```python
from build123d import *

# Parameters (mm, degrees)
SHELL1_T = -0.75


with BuildPart() as part:
    # Sketch1 → Revolve1 (revolve)
    with BuildSketch(Plane(origin=(0, 0, 0), x_dir=(1, 0, 0), z_dir=(0, 1, 0)), mode=Mode.PRIVATE) as revolve1_sk:
        Polygon((3.5, 16.5), (3.5, -16.5), (2.5, -16.5), (2.5, -19.5), (0, -19.5), (0, -16.5), (0, 16.5), (0, 19.5), (2.5, 19.5), (2.5, 16.5), align=None)
    revolve(revolve1_sk.sketch.rotate(Axis((0, 0, -21.376645948), (0, 0, 1)), 180), axis=Axis((0, 0, -21.376645948), (0, 0, 1)))

    # Shell1
    shell1_openings = [part.faces().sort_by_distance(p)[0] for p in [
        (0, 0, -19.5),
        (0, 0, 19.5),
    ]]
    offset(amount=SHELL1_T, openings=shell1_openings, kind=Kind.INTERSECTION)


solid = part.part
```
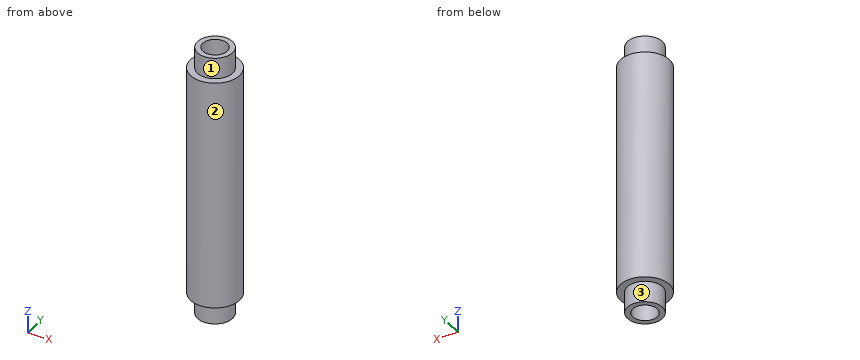
The model under review builds one solid part; all positions refer to its coordinate system, in mm. Face numbers are marked on the shaded views. A direction names the side the tool comes from. Round coordinates to 2 decimals unless told otherwise and drop trailing zeros. Write each loop counter-clockwise with the first axis right and the second up, starting at its lowest first coordinate (ties: lowest second). Pieces come first, ordered by that corner, then holes. Notation, with made-up numbers: M -2.5,62.5 L 13.5,62.5 A12 cw 13.5,85.5 Z; hole C 17,24 d10. An arc over 180 degrees is marked long. Use CSV: the item, a comma, the result in double quotes. Start each with the question number.
(1) For line 1 along Y through (x, z) = (0, -17.75); line 2 along Z through (x, y) = (-1.5, 1.25); line 3 along Y through (x, z) = (0, 7.5), list the stretches that pass through material, from the lowest coordinate up.
(2) Tool access review of the marked faces 1, 2 and 3: name each direction out of +Z, -Z, +X, -X, +Y, -Y from which nothing blocks a thin tool from reaching the whole face with its end or side.
(3) We need section C-C, the plane z = 6.5. State the section outline as (x, y) points, then the cut area to 3 significant figures.
(4) We need section A-A, the plane y = 0. State the section outline as (x, z) points.
Findings:
1,line 1,"-2.5 to -1.75, 1.75 to 2.5"
1,line 2,"-19.5 to -15.75, 15.75 to 19.5"
1,line 3,"-3.5 to -2.75, 2.75 to 3.5"
2,face 1,"+Z"
2,face 2,"+Z, -Z"
2,face 3,"-Z"
3,outline,"C 0,0 d7; hole C 0,0 d5.5"
3,area,"14.7 mm^2"
4,outline,"M -3.5,-16.5 L -2.5,-16.5 L -2.5,-19.5 L -1.75,-19.5 L -1.75,-15.75 L -2.75,-15.75 L -2.75,15.75 L -1.75,15.75 L -1.75,19.5 L -2.5,19.5 L -2.5,16.5 L -3.5,16.5 Z; M 1.75,-19.5 L 2.5,-19.5 L 2.5,-16.5 L 3.5,-16.5 L 3.5,16.5 L 2.5,16.5 L 2.5,19.5 L 1.75,19.5 L 1.75,15.75 L 2.75,15.75 L 2.75,-15.75 L 1.75,-15.75 Z"
